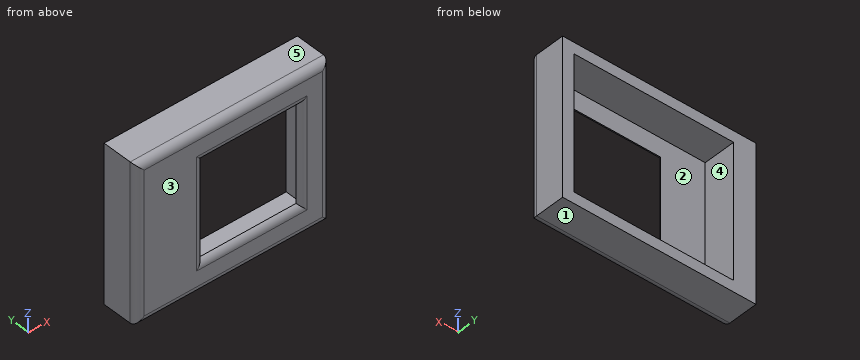
from build123d import *

# Parameters (mm, degrees)
F0_W         = 52
F0_H         = 42
F1_DEPTH     = 10
F2_W         = 26
F2_H         = 26
F3_DEPTH     = 25
F4_W         = 43
F4_H         = 36
F4_W_2       = 26
F4_H_2       = 26
F5_DEPTH     = 8.7
F6_T1_DEPTH  = 52
F6_T3_DEPTH  = 62
F6_T5_DEPTH  = 26
F6_T7_DEPTH  = 26
F6_T13_DEPTH = 30.6837484988
F6_T17_DEPTH = 30.6837484988
F6_T24_DEPTH = 30.6837484988
F6_T28_DEPTH = 30.6837484988
F6_T35_DEPTH = 30.6837484988
F6_T39_DEPTH = 30.6837484988
F6_T46_DEPTH = 30.6837484988
F6_T50_DEPTH = 30.6837484988


# Not quite as in the source:
# - a fillet or chamfer that OpenCascade refuses, or shapes differently, is made with other operations: its cross-section is extruded or revolved along the edge and cut away or added


with BuildPart() as f1:
    # F0 (on Front) → F1 (new body)
    with BuildSketch(Plane.XZ):
        Rectangle(F0_W, F0_H)
    extrude(amount=-F1_DEPTH)

    # F2 (on face) → F3 (cut)
    with BuildSketch(Plane.XZ):
        with Locations((5, 0)):
            Rectangle(F2_W, F2_H)
    extrude(amount=-F3_DEPTH, mode=Mode.SUBTRACT)

    # F4 (on face) → F5 (cut)
    with BuildSketch(Plane(origin=(0, 10, 0), x_dir=(-1, 0, 0), z_dir=(0, 1, 0))):
        with Locations((-1.5, 0)):
            Rectangle(F4_W, F4_H)
        with Locations((-5, 0)):
            Rectangle(F4_W_2, F4_H_2, mode=Mode.SUBTRACT)
    extrude(amount=-F5_DEPTH, mode=Mode.SUBTRACT)

    # F6: fillet of radius 2 on 8 edges, made by hand

    # F6_s2 → F6_t1 (cut)
    with BuildSketch(Plane.XY.offset(-26)):
        with BuildLine():
            ThreePointArc((-26, 2), (-25.4142135624, 0.5857864376), (-24, 0))
            Line((-24, 0), (-26, 0))
            Line((-26, 0), (-26, 2))
        make_face()
        with BuildLine():
            ThreePointArc((26, 2), (25.4142135624, 0.5857864376), (24, 0))
            Line((24, 0), (26, 0))
            Line((26, 0), (26, 2))
        make_face()
    extrude(amount=F6_T1_DEPTH, mode=Mode.SUBTRACT)

    # F6_s4 → F6_t3 (cut)
    with BuildSketch(Plane.YZ.offset(-31)):
        with BuildLine():
            ThreePointArc((0, 19), (0.5857864376, 20.4142135624), (2, 21))
            Line((2, 21), (0, 21))
            Line((0, 21), (0, 19))
        make_face()
        with BuildLine():
            ThreePointArc((2, -21), (0.5857864376, -20.4142135624), (0, -19))
            Line((0, -19), (0, -21))
            Line((0, -21), (2, -21))
        make_face()
    extrude(amount=F6_T3_DEPTH, mode=Mode.SUBTRACT)

    # F6_s6 → F6_t5 (cut)
    with BuildSketch(Plane.XY.offset(-13)):
        with BuildLine():
            ThreePointArc((-9.8734993995, 0), (-8.7333239744, 0.3568323275), (-8, 1.3))
            Line((-8, 1.3), (-8, 0))
            Line((-8, 0), (-9.8734993995, 0))
        make_face()
        with BuildLine():
            ThreePointArc((19.8734993995, 0), (18.7333239744, 0.3568323275), (18, 1.3))
            Line((18, 1.3), (18, 0))
            Line((18, 0), (19.8734993995, 0))
        make_face()
    extrude(amount=F6_T5_DEPTH, mode=Mode.SUBTRACT)

    # F6_s8 → F6_t7 (cut)
    with BuildSketch(Plane.YZ.offset(-8)):
        with BuildLine():
            ThreePointArc((0, -14.8734993995), (0.3568323275, -13.7333239744), (1.3, -13))
            Line((1.3, -13), (0, -13))
            Line((0, -13), (0, -14.8734993995))
        make_face()
        with BuildLine():
            ThreePointArc((0, 14.8734993995), (0.3568323275, 13.7333239744), (1.3, 13))
            Line((1.3, 13), (0, 13))
            Line((0, 13), (0, 14.8734993995))
        make_face()
    extrude(amount=F6_T7_DEPTH, mode=Mode.SUBTRACT)


with BuildPart() as f6_tool11:
    # F6_s12 → F6_t13 (new body)
    with BuildSketch(Plane.YZ.offset(18)):
        with BuildLine():
            ThreePointArc((0, 14.8734993995), (0.3568323275, 13.7333239744), (1.3, 13))
            Line((1.3, 13), (0, 13))
            Line((0, 13), (0, 14.8734993995))
        make_face()
    extrude(amount=-F6_T13_DEPTH)

    split(bisect_by=Plane.YZ.offset(-8), keep=Keep.BOTTOM)


with BuildPart() as f6_tool15:
    # F6_s16 → F6_t17 (new body)
    with BuildSketch(Plane.XY.offset(17.6837484988)):
        with BuildLine():
            ThreePointArc((-9.8734993995, 0), (-8.7333239744, 0.3568323275), (-8, 1.3))
            Line((-8, 1.3), (-8, 0))
            Line((-8, 0), (-9.8734993995, 0))
        make_face()
    extrude(amount=-F6_T17_DEPTH)

    split(bisect_by=Plane.XY.offset(13), keep=Keep.TOP)


with BuildPart() as f6_tool11_1:
    add(f6_tool11.part)

    # F6_t19: intersect F6_tool15
    add(f6_tool15.part, mode=Mode.INTERSECT)


with BuildPart() as f1_1:
    add(f1.part)

    # F6_t9: cut F6_tool11
    add(f6_tool11_1.part, mode=Mode.SUBTRACT)


with BuildPart() as f6_tool22:
    # F6_s23 → F6_t24 (new body)
    with BuildSketch(Plane.XY.offset(13)):
        with BuildLine():
            ThreePointArc((-9.8734993995, 0), (-8.7333239744, 0.3568323275), (-8, 1.3))
            Line((-8, 1.3), (-8, 0))
            Line((-8, 0), (-9.8734993995, 0))
        make_face()
    extrude(amount=-F6_T24_DEPTH)

    split(bisect_by=Plane.XY.offset(-13), keep=Keep.BOTTOM)


with BuildPart() as f6_tool26:
    # F6_s27 → F6_t28 (new body)
    with BuildSketch(Plane.YZ.offset(-12.6837484988)):
        with BuildLine():
            ThreePointArc((0, -14.8734993995), (0.3568323275, -13.7333239744), (1.3, -13))
            Line((1.3, -13), (0, -13))
            Line((0, -13), (0, -14.8734993995))
        make_face()
    extrude(amount=F6_T28_DEPTH)

    split(bisect_by=Plane.YZ.offset(-8), keep=Keep.BOTTOM)


with BuildPart() as f6_tool22_1:
    add(f6_tool22.part)

    # F6_t30: intersect F6_tool26
    add(f6_tool26.part, mode=Mode.INTERSECT)


with BuildPart() as f1_2:
    add(f1_1.part)

    # F6_t20: cut F6_tool22
    add(f6_tool22_1.part, mode=Mode.SUBTRACT)


with BuildPart() as f6_tool33:
    # F6_s34 → F6_t35 (new body)
    with BuildSketch(Plane.XY.offset(-17.6837484988)):
        with BuildLine():
            ThreePointArc((19.8734993995, 0), (18.7333239744, 0.3568323275), (18, 1.3))
            Line((18, 1.3), (18, 0))
            Line((18, 0), (19.8734993995, 0))
        make_face()
    extrude(amount=F6_T35_DEPTH)

    split(bisect_by=Plane.XY.offset(-13), keep=Keep.BOTTOM)


with BuildPart() as f6_tool37:
    # F6_s38 → F6_t39 (new body)
    with BuildSketch(Plane.YZ.offset(-8)):
        with BuildLine():
            ThreePointArc((0, -14.8734993995), (0.3568323275, -13.7333239744), (1.3, -13))
            Line((1.3, -13), (0, -13))
            Line((0, -13), (0, -14.8734993995))
        make_face()
    extrude(amount=F6_T39_DEPTH)

    split(bisect_by=Plane.YZ.offset(18), keep=Keep.TOP)


with BuildPart() as f6_tool33_1:
    add(f6_tool33.part)

    # F6_t41: intersect F6_tool37
    add(f6_tool37.part, mode=Mode.INTERSECT)


with BuildPart() as f1_3:
    add(f1_2.part)

    # F6_t31: cut F6_tool33
    add(f6_tool33_1.part, mode=Mode.SUBTRACT)


with BuildPart() as f6_tool44:
    # F6_s45 → F6_t46 (new body)
    with BuildSketch(Plane.XY.offset(-13)):
        with BuildLine():
            ThreePointArc((19.8734993995, 0), (18.7333239744, 0.3568323275), (18, 1.3))
            Line((18, 1.3), (18, 0))
            Line((18, 0), (19.8734993995, 0))
        make_face()
    extrude(amount=F6_T46_DEPTH)

    split(bisect_by=Plane.XY.offset(13), keep=Keep.TOP)


with BuildPart() as f6_tool48:
    # F6_s49 → F6_t50 (new body)
    with BuildSketch(Plane.YZ.offset(22.6837484988)):
        with BuildLine():
            ThreePointArc((0, 14.8734993995), (0.3568323275, 13.7333239744), (1.3, 13))
            Line((1.3, 13), (0, 13))
            Line((0, 13), (0, 14.8734993995))
        make_face()
    extrude(amount=-F6_T50_DEPTH)

    split(bisect_by=Plane.YZ.offset(18), keep=Keep.TOP)


with BuildPart() as f6_tool44_1:
    add(f6_tool44.part)

    # F6_t52: intersect F6_tool48
    add(f6_tool48.part, mode=Mode.INTERSECT)


with BuildPart() as f1_4:
    add(f1_3.part)

    # F6_t42: cut F6_tool44
    add(f6_tool44_1.part, mode=Mode.SUBTRACT)


solid = f1_4.part
Here's how the part is built. I have some questions about the finished solid (model axes, mm). Face numbers are marked on the shaded views. A direction names the side the tool comes from. Give positions to 0.01 mm unless a question says otherwise; leave off trailing zeros. Order: outer loops, then holes, each group sorted by start corner. A loop starts at its lowest first (then second) coordinate and runs counter-clockwise, first axis right, second up. Notation, with made-up numbers: (3.25, 40.25) -> (56.25, 40.25) arc R17 cw to (56.25, 63.25) -> close; hole circle Ø4 at (-13.5, 82). An arc over 180 degrees is marked (long way). One line per item, written item: value. Start each with the question number.
1. Imagine slicing it at B-B, the plane z = 11. List the corners of the cut face in (x, y) for me, plus the area to 3 significant figures.
2. For the marked faces 1 and 2, which set-ups out of +Z, -Z, +X, -X, +Y, -Y let a thin tool reach every point of the face, with its end or its side?
3. Imagine slicing it at A-A, the plane y = 7. List the corners of the cut face in (x, z) for me, plus the area to 3 significant figures.
4. We'd pull the mould along Z, two halves only. Please class the marked faces 3, 4 and 5: released by +Z, released by -Z, zero draft, split by the parting line, or undercut.
5. Imagine slicing it at D-D, the plane x = -12. List the corners of the cut face in (y, z) for me, plus the area to 3 significant figures.
6. Imagine slicing it at C-C, the plane x = 11.5. List the corners of the cut face in (y, z) for me.
7. Will this pin go through, and if not, where does the flat tip stop? pin 1 Ø4 at (x, z) = (0, 12.5) entering from +Y.
8. I need wall thicknesses on probe 1 along X at (y, z) = (3.75, -13.5); probe 2 along Z at (x, y) = (-13.5, 4.75); probe 3 along Y at (x, z) = (-10, 15.5). Which ranges of each line are inside material? Lowest first, please. Write a range as from..to.
Values follow:
1. outline: (-26, 2) arc R2 ccw to (-24, 0) -> (-9.87, 0) arc R2 ccw to (-8, 1.3) -> (-20, 1.3) -> (-20, 10) -> (-26, 10) -> close; (18, 1.3) arc R2 ccw to (19.87, 0) -> (24, 0) arc R2 ccw to (26, 2) -> (26, 10) -> (23, 10) -> (23, 1.3) -> close
1. area: 109 mm2
2. face 1: -Z, +X, -X, +Y, -Y
2. face 2: +Y
3. outline: (-26, -21) -> (26, -21) -> (26, 21) -> (-26, 21) -> close; hole (-20, -18) -> (23, -18) -> (23, 18) -> (-20, 18) -> close
3. area: 636 mm2
4. face 3: zero draft
4. face 4: undercut
4. face 5: released by +Z
5. outline: (0, -19) arc R2 ccw to (2, -21) -> (10, -21) -> (10, -18) -> (1.3, -18) -> (1.3, 18) -> (10, 18) -> (10, 21) -> (2, 21) arc R2 ccw to (0, 19) -> close
5. area: 105 mm2
6. outline: (0, -19) arc R2 ccw to (2, -21) -> (10, -21) -> (10, -18) -> (1.3, -18) -> (1.3, -13) arc R2 ccw to (0, -14.87) -> close; (0, 14.87) arc R2 ccw to (1.3, 13) -> (1.3, 18) -> (10, 18) -> (10, 21) -> (2, 21) arc R2 ccw to (0, 19) -> close
7. pin 1: stops at y = 1.3
8. probe 1: x = -26..-20, 23..26
8. probe 2: z = -21..-18, 18..21
8. probe 3: y = 0..1.3
